from build123d import *

# Parameters (mm, degrees)
SKETCH1_R           = 5.334
BOSS_EXTRUDE1_DEPTH = 11.90625


with BuildPart() as part:
    # Sketch1 → Boss-Extrude1 (new body)
    with BuildSketch(Plane.XY):
        Polygon((0, 0), (0, 302.324826907), (388.9375, 574.661796299), (388.9375, 272.336969392), align=None)
        with Locations((19.05, 292.408024594)):
            Circle(SKETCH1_R, mode=Mode.SUBTRACT)
        with Locations((19.05, 36.594709519)):
            Circle(SKETCH1_R, mode=Mode.SUBTRACT)
        with Locations((369.8875, 282.253771705)):
            Circle(SKETCH1_R, mode=Mode.SUBTRACT)
        with Locations((369.8875, 538.06708678)):
            Circle(SKETCH1_R, mode=Mode.SUBTRACT)
    extrude(amount=BOSS_EXTRUDE1_DEPTH)


solid = part.part
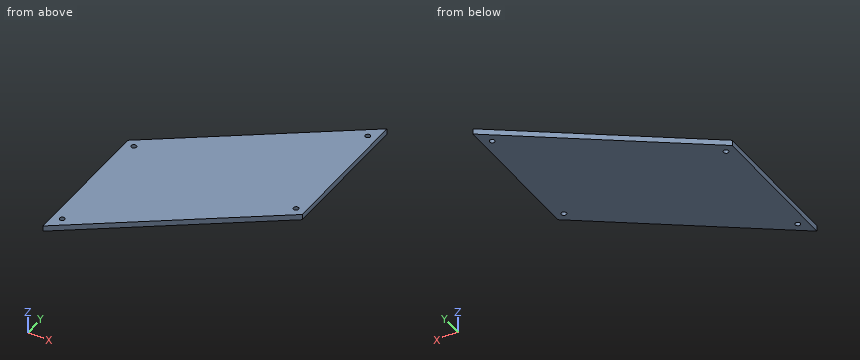
Model file for the job. Use its own axes, mm. Give positions to 0.01 mm unless a question says otherwise; leave off trailing zeros. Loops run counter-clockwise (first coordinate to the right, second up) from the corner with the lowest first, then second, coordinate; pieces in that order, holes last.
Item 1: Drill centre lines: line 1 along Y through (x, z) = (368, 10.75); line 2 along X through (y, z) = (285, 4.5); line 3 along X through (y, z) = (37, 6.5). Where is each one in solid material? Low to high.
Check values:
line 1: y = 257.68 to 277.26, 287.24 to 533.08, 543.06 to 560
line 2: x = 0 to 365.31, 374.46 to 388.94
line 3: x = 0 to 13.73, 24.37 to 52.84
Item 2: Drop flat-ended pins along their axis: P1, Ø5, axis at x = 160, z = 10.5, coming from the +Y side; P2, Ø1, axis at x = 213.5, z = 5.5, coming from the +Y side. Give the stop position or say it passes through.
Check values:
P1: stops at y = 416.11
P2: stops at y = 452.17
Item 3: Slice it at C-C (y = 406.5). Write the cut outline in (x, z).
Check values:
outline: (148.78, 0) - (388.94, 0) - (388.94, 11.91) - (148.78, 11.91) - close
Item 4: Slice it at A-A (z = 9.25). Write the cut outline in (x, y).
Check values:
outline: (0, 0) - (388.94, 272.34) - (388.94, 574.66) - (0, 302.32) - close; hole circle Ø10.67 at (19.05, 36.59); hole circle Ø10.67 at (19.05, 292.41); hole circle Ø10.67 at (369.89, 282.25); hole circle Ø10.67 at (369.89, 538.07)
Item 5: Slice it at B-B (x = 128). Write the cut outline in (y, z).
Check values:
outline: (89.63, 0) - (391.95, 0) - (391.95, 11.91) - (89.63, 11.91) - close
